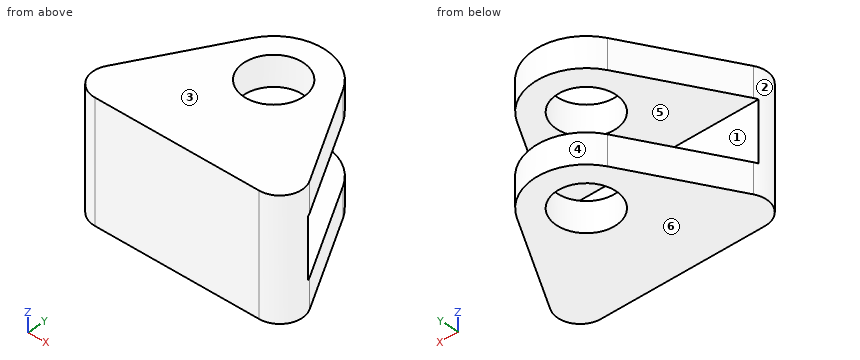
from build123d import *

# Parameters (mm, degrees)
SKETCH1_R           = 4
MAINBODY_DEPTH      = 4
BOSS_EXTRUDE2_DEPTH = 8
FILLET1_R           = 3


with BuildPart() as part:
    # Sketch1 → MainBody (new body)
    with BuildSketch(Plane.XY):
        with BuildLine():
            Line((-6.062177826, 3.5), (-16.165807537, -14))
            Line((-16.165807537, -14), (16.165807537, -14))
            Line((16.165807537, -14), (6.062177826, 3.5))
            ThreePointArc((6.062177826, 3.5), (0, 7), (-6.062177826, 3.5))
        make_face()
        Circle(SKETCH1_R, mode=Mode.SUBTRACT)
    mainbody = extrude(amount=MAINBODY_DEPTH)

    # Sketch3 → Boss-Extrude2 (add)
    with BuildSketch(Plane(origin=(0, 0, 0), x_dir=(-1, 0, 0), z_dir=(0, 0, -1))):
        Polygon((-16.165807537, -14), (-13.856406461, -10), (13.856406461, -10), (16.165807537, -14), align=None)
    extrude(amount=BOSS_EXTRUDE2_DEPTH)

    # Mirror2: MainBody across plane
    add(mainbody.mirror(Plane(origin=(0, 0, -4), x_dir=(1, 0, 0), z_dir=(0, 0, -1))))

    # Fillet1
    # the kernel refuses this fillet: 3 mm, written as the material it takes off along each edge
    with BuildSketch(Plane(origin=(-16.165807537, -14, -24.990381057), x_dir=(1, 0, 0), z_dir=(0, 0, 1)), Plane(origin=(16.165807537, -14, 16.990381057), x_dir=(-1, 0, 0), z_dir=(0, 0, -1))) as fillet1_piece_1:
        with BuildLine():
            CenterArc((FILLET1_R * 1.73205080757, FILLET1_R), FILLET1_R, 150, 120)
            Line((FILLET1_R * 0.866025403784, FILLET1_R * 1.5), (0, 0))
            Line((0, 0), (FILLET1_R * 1.73205080757, 0))
        make_face()
    extrude(amount=41.980762114, mode=Mode.SUBTRACT)


solid = part.part
Design review of the part built by this model. Coordinates are the model's own, in mm. Face numbers are marked on the shaded views. A direction names the side the tool comes from. Give positions to 0.01 mm unless a question says otherwise; leave off trailing zeros. Order: outer loops, then holes, each group sorted by start corner. A loop starts at its lowest first (then second) coordinate and runs counter-clockwise, first axis right, second up. Notation, with made-up numbers: (62.25, -19) - (114.25, -19) arc R14 ccw to (114.25, -7) - close; hole circle Ø4 at (-15, 18). An arc over 180 degrees is marked (long way). Write item = value, one per line. Start each with the question number.
Q1. We need section A-A on x = 0. State the section outline as (y, z) points.
Q2. Tool access review of the marked faces 1 and 2: name each direction out of +Z, -Z, +X, -X, +Y, -Y from which nothing blocks a thin tool from reaching the whole face with its end or side.
Q3. Mouldability with a two-part tool opening along Z and no side actions: class the marked faces 3, 4, 5 and 6 as released by +Z, released by -Z, zero draft, split by the parting line, or undercut.
Q4. We need section D-D on y = 0. State the section outline as (x, z) points, plus the area to 3 significant figures.
Q5. We need section B-B on y = 5.25. State the section outline as (x, z) points, plus the area to 3 significant figures.
Q6. Clearance check with flat-ended pins moving along their axes: pin 1 Ø6 at (x, z) = (-3.5, 0) entering from +Y; pin 2 Ø4 at (x, z) = (-6.5, 0.5) entering from +Y. State where each tip first meets the part, or that it passes through.
Q7. To check wall thickness, follow L1, parallel to Z at x = 10.75, y = -8; L2, parallel to Y at x = 7, z = -2.75; L3, parallel to X at y = 3.5, z = 3. State the ranges of each line that lie inside material, in increasing order. Write a range as from..to.
Q8. We need section C-C on z = -9. State the section outline as (x, y) points, plus the area to 3 significant figures.
Working result:
q1.outline = (-14, -12) - (-4, -12) - (-4, -8) - (-10, -8) - (-10, 0) - (-4, 0) - (-4, 4) - (-14, 4) - close; (4, -12) - (7, -12) - (7, -8) - (4, -8) - close; (4, 0) - (7, 0) - (7, 4) - (4, 4) - close
q2.face_1 = +X, -X, +Y
q2.face_2 = +Z, -Z, -X
q3.face_3 = released by +Z
q3.face_4 = zero draft
q3.face_5 = undercut
q3.face_6 = released by -Z
q4.outline = (-8.08, -12) - (-4, -12) - (-4, -8) - (-8.08, -8) - close; (-8.08, 0) - (-4, 0) - (-4, 4) - (-8.08, 4) - close; (4, -12) - (8.08, -12) - (8.08, -8) - (4, -8) - close; (4, 0) - (8.08, 0) - (8.08, 4) - (4, 4) - close
q4.area = 65.3 mm²
q5.outline = (-4.63, -12) - (4.63, -12) - (4.63, -8) - (-4.63, -8) - close; (-4.63, 0) - (4.63, 0) - (4.63, 4) - (-4.63, 4) - close
q5.area = 74.1 mm²
q6.pin_1 = 6.98
q6.pin_2 = 5.36
q7.L1 = -12..-8, 0..4
q7.L2 = -14..-10
q7.L3 = -6.06..-1.94, 1.94..6.06
q8.outline = (-13.57, -9.5) arc R3 ccw to (-10.97, -14) - (10.97, -14) arc R3 ccw to (13.57, -9.5) - (6.06, 3.5) arc R7 ccw to (-6.06, 3.5) - close; hole circle Ø8 at (0, 0)
q8.area = 356 mm²
